Check sheet for the modelled part. Datum: model origin and axes. Units: mm. A direction names the side the tool comes from. Give positions to 0.01 mm unless a question says otherwise; leave off trailing zeros. Write each loop counter-clockwise with the first axis right and the second up, starting at its lowest first coordinate (ties: lowest second). Pieces come first, ordered by that corner, then holes. Notation, with made-up numbers: (23, 54) -> (49, 54) arc R25 cw to (49, 88) -> close; hole circle Ø6 at (64.25, 3.5). An arc over 180 degrees is marked (long way). Answer as a JSON object with one key per item and string values.
from build123d import *

# Parameters (mm, degrees)
SKETCH2_W                 = 150
SKETCH2_H                 = 300
BOXPLATFORM_DEPTH         = 7.5
SKETCH3_W                 = 80
SKETCH3_H                 = 60
EXTRUSIONCONNECTION_DEPTH = 20
FILLET1_R                 = 10
MOUNTSLOTS_DEPTH          = 444.962367113
WASHERSLOTS_DEPTH         = 20
SKETCH7_W                 = 7.3
SKETCH7_H                 = 60
WALLS_DEPTH               = 101.2
FILLET2_R                 = 10
FILLET3_R                 = 10
SKETCH8_R                 = 2
M3X7MMHOLES_DEPTH         = 8


with BuildPart() as part:
    # Sketch2 → BoxPlatform (new body)
    with BuildSketch(Plane.XY):
        with Locations((-9.387993296, -285)):
            Rectangle(SKETCH2_W, SKETCH2_H)
    extrude(amount=BOXPLATFORM_DEPTH)

    # Sketch3 → ExtrusionConnection (add)
    with BuildSketch(Plane.XY.offset(7.5)):
        with Locations((-9.387993296, -285)):
            Rectangle(SKETCH3_W, SKETCH3_H)
    extrude(amount=EXTRUSIONCONNECTION_DEPTH)

    # Fillet1
    fillet1_edges = [part.edges().sort_by_distance(p)[0] for p in [
        (-9.387993296, -315, 7.5),
        (30.612006704, -285, 7.5),
        (-9.387993296, -255, 7.5),
        (-49.387993296, -285, 7.5),
    ]]
    fillet(fillet1_edges, radius=FILLET1_R)

    # Sketch5 → MountSlots (cut, through all)
    with BuildSketch(Plane.XY.offset(27.5)):
        with BuildLine():
            Line((17.612006704, -305), (17.612006704, -265))
            ThreePointArc((17.612006704, -265), (20.612006704, -262), (23.612006704, -265))
            Line((23.612006704, -265), (23.612006704, -305))
            ThreePointArc((23.612006704, -305), (20.612006704, -308), (17.612006704, -305))
        make_face()
        with BuildLine():
            Line((-42.387993296, -305), (-42.387993296, -265))
            ThreePointArc((-42.387993296, -265), (-39.387993296, -262), (-36.387993296, -265))
            Line((-36.387993296, -265), (-36.387993296, -305))
            ThreePointArc((-36.387993296, -305), (-39.387993296, -308), (-42.387993296, -305))
        make_face()
        with BuildLine():
            Line((-12.387993296, -305), (-12.387993296, -265))
            ThreePointArc((-12.387993296, -265), (-9.387993296, -262), (-6.387993296, -265))
            Line((-6.387993296, -265), (-6.387993296, -305))
            ThreePointArc((-6.387993296, -305), (-9.387993296, -308), (-12.387993296, -305))
        make_face()
    extrude(amount=-MOUNTSLOTS_DEPTH, mode=Mode.SUBTRACT)

    # Sketch6 → WasherSlots (cut)
    with BuildSketch(Plane(origin=(0, 0, 0), x_dir=(-1, 0, 0), z_dir=(0, 0, -1))):
        with BuildLine():
            Line((-15.612006704, -265), (-15.612006704, -305))
            ThreePointArc((-15.612006704, -305), (-20.612006704, -310), (-25.612006704, -305))
            Line((-25.612006704, -305), (-25.612006704, -265))
            ThreePointArc((-25.612006704, -265), (-20.612006704, -260), (-15.612006704, -265))
        make_face()
        with BuildLine():
            Line((14.387993296, -265), (14.387993296, -305))
            ThreePointArc((14.387993296, -305), (9.387993296, -310), (4.387993296, -305))
            Line((4.387993296, -305), (4.387993296, -265))
            ThreePointArc((4.387993296, -265), (9.387993296, -260), (14.387993296, -265))
        make_face()
        with BuildLine():
            Line((44.387993296, -265), (44.387993296, -305))
            ThreePointArc((44.387993296, -305), (39.387993296, -310), (34.387993296, -305))
            Line((34.387993296, -305), (34.387993296, -265))
            ThreePointArc((34.387993296, -265), (39.387993296, -260), (44.387993296, -265))
        make_face()
    extrude(amount=-WASHERSLOTS_DEPTH, mode=Mode.SUBTRACT)

    # Sketch7 → Walls (add)
    with BuildSketch(Plane(origin=(0, 0, 0), x_dir=(-1, 0, 0), z_dir=(0, 0, -1))):
        Polygon((64.587993296, -135), (84.387993296, -135), (84.387993296, -154.8), (77.087993296, -154.8), (77.087993296, -142.3), (64.587993296, -142.3), align=None)
        Polygon((84.387993296, -435), (84.387993296, -415.2), (77.087993296, -415.2), (77.087993296, -427.7), (64.587993296, -427.7), (64.587993296, -435), align=None)
        Polygon((-45.812006704, -142.3), (-58.312006704, -142.3), (-58.312006704, -154.8), (-65.612006704, -154.8), (-65.612006704, -135), (-45.812006704, -135), align=None)
        Polygon((-65.612006704, -435), (-65.612006704, -415.2), (-58.312006704, -415.2), (-58.312006704, -427.7), (-45.812006704, -427.7), (-45.812006704, -435), align=None)
        with Locations((-61.962006704, -326.5)):
            Rectangle(SKETCH7_W, SKETCH7_H)
        with Locations((80.737993296, -326.5)):
            Rectangle(SKETCH7_W, SKETCH7_H)
    extrude(amount=WALLS_DEPTH)

    # Fillet2
    fillet2_edges = [part.edges().sort_by_distance(p)[0] for p in [
        (65.612006704, -435, -46.85),
        (-84.387993296, -435, -46.85),
        (-84.387993296, -135, -46.85),
        (65.612006704, -135, -46.85),
    ]]
    fillet(fillet2_edges, radius=FILLET2_R)

    # Fillet3
    fillet3_edges = [part.edges().sort_by_distance(p)[0] for p in [
        (-64.587993296, -138.65, 0),
        (-80.737993296, -154.8, 0),
        (-80.737993296, -415.2, 0),
        (-64.587993296, -431.35, 0),
        (61.962006704, -154.8, 0),
        (45.812006704, -138.65, 0),
        (61.962006704, -415.2, 0),
        (45.812006704, -431.35, 0),
        (61.962006704, -356.5, 0),
        (61.962006704, -296.5, 0),
        (-80.737993296, -296.5, 0),
        (-80.737993296, -356.5, 0),
    ]]
    fillet(fillet3_edges, radius=FILLET3_R)

    # Sketch8 → M3x7mmHoles (cut)
    with BuildSketch(Plane(origin=(0, 0, -101.2), x_dir=(-1, 0, 0), z_dir=(0, 0, -1))):
        with Locations((80.887993296, -147.8)):
            Circle(SKETCH8_R)
        with Locations((-61.812006704, -147.8)):
            Circle(SKETCH8_R)
        with Locations((80.887993296, -326.5)):
            Circle(SKETCH8_R)
        with Locations((-61.812006704, -326.5)):
            Circle(SKETCH8_R)
        with Locations((80.887993296, -422.2)):
            Circle(SKETCH8_R)
        with Locations((-61.812006704, -422.2)):
            Circle(SKETCH8_R)
    extrude(amount=-M3X7MMHOLES_DEPTH, mode=Mode.SUBTRACT)


solid = part.part
1. Sectioned sample at A-A, the plane z = -24.5. State how many separate pieces and enclosed holes the cut face has, plus the area to 3 significant figures.
Determined:
{"separate pieces": "6", "enclosed holes": "0", "area": "1,730 mm^2"}
2. Sectioned sample at C-C, the plane y = -223. Enter the section's corners in (x, z), plus the area to 4 significant figures.
Determined:
{"outline": "(-84.39, 0) -> (65.61, 0) -> (65.61, 7.5) -> (-84.39, 7.5) -> close", "area": "1,125 mm^2"}
3. Mould release check, pull along Y, two halves, no side actions. Record for faces 1 (the face through (-64.588, -139, -55)), 2 (the face through (-8.69, -318.01, 10.35)), 3 (the face through (-71, -427.7, -50)): released by +Y, released by -Y, zero draft, split by the parting line, or undercut.
Determined:
{"face 1": "zero draft", "face 2": "released by -Y", "face 3": "undercut"}
4. Go/stop test with flat-tipped pins: P1, Ø8, axis at y = -256, z = -4.5, coming from the -X side; P2, Ø2, axis at x = -82.5, z = -69, coming from the +Y side; P3, Ø3, axis at x = -81, y = -423, coming from the -Z side; P4, Ø3, axis at x = -56, y = -345.5, coming from the +Z side. Record where each tip stops, or that it passes through.
Determined:
{"P1": "through", "P2": "y = -137.97", "P3": "z = -101.2", "P4": "z = 7.5"}
5. Access from +Z, -Z, +X, -X, +Y, -Y to the whole of each face (thin tool, end or side, straight path). Record for faces 4 (the face through (-12.388, -285, 24)), 5 (the face through (-84.388, -305, -43)), 6 (the face through (-80.79, -293.49, -2.85)), 7 (the face through (-44.388, -285, 10)), 8 (the face through (42.805, -431.401, -2.852)).
Determined:
{"face 4": "+Z, -Z", "face 5": "+Z, -Z, -X, +Y, -Y", "face 6": "-Z, +X, -X", "face 7": "-Z", "face 8": "-Z, +Y, -Y"}
6. Scan lines: L1, parallel to X at y = -422.2, z = -97.75; L2, parallel to X at y = -350, z = -11; L3, parallel to Y at x = 50, z = -80. Record each from-to range of solid material in increasing order. Write a range as [from, to].
Determined:
{"L1": "[-84.39, -82.89], [-78.89, -77.09], [58.31, 59.81], [63.81, 65.61]", "L2": "[-84.39, -77.09], [58.31, 65.61]", "L3": "[-435, -427.7], [-142.3, -135]"}
